The drawing under review shows one solid part. Ordinate dimensions are in mm from its lowest x, y, z. A direction names the side the tool comes from. Give positions to 0.01 mm unless a question says otherwise; leave off trailing zeros. Order: outer loops, then holes, each group sorted by start corner. A loop starts at its lowest first (then second) coordinate and runs counter-clockwise, first axis right, second up. Notation, with made-up numbers: (44, 39) - (102, 39) arc R17 ccw to (102, 51) - close; hole circle Ø9 at (-8, 12). An arc over 180 degrees is marked (long way). Use CSV: the item, a comma, the result in double quotes. Start each with the question number.
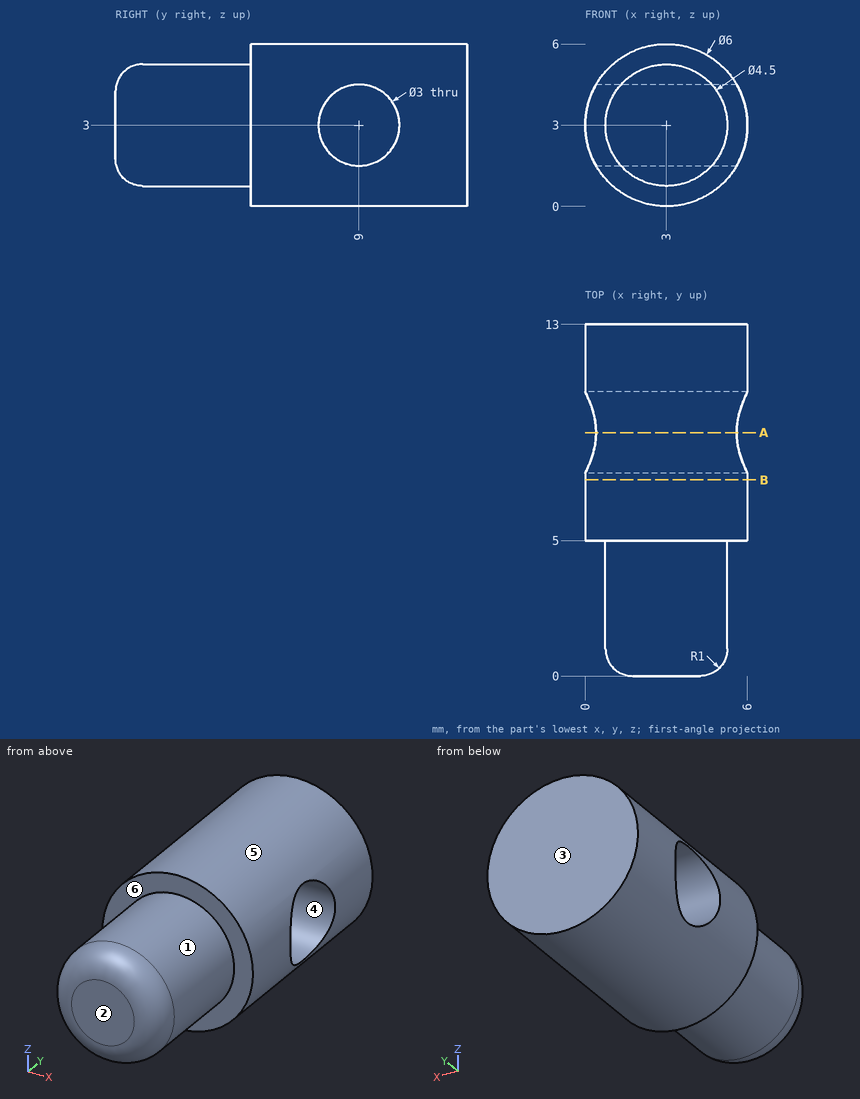
1. Clearance check with flat-ended pins moving along their axes: pin 1 (1 mm diameter, centred on x = 1, y = 6.5, fed in from -Z); pin 2 (2 mm diameter, centred on y = 9, z = 5, fed in from -X); pin 3 (1.5 mm diameter, centred on y = 8, z = 5, fed in from +X). State where each tip first meets the part, or that it passes through.
2. To check wall thickness, follow L1, parallel to Y at x = 3.5, z = 3; L2, parallel to Z at x = 3, y = 9; L3, parallel to X at y = 3, z = 3. State the ranges of each line that lie inside material, in increasing order. Write a range as [from, to].
3. Tool access review of the marked faces 5 and 6: name each direction out of +Z, -Z, +X, -X, +Y, -Y from which nothing blocks a thin tool from reaching the whole face with its end or side.
4. Mouldability with a two-part tool opening along Y and no side actions: class the marked faces 1, 2, 3 and 4 as pulls with the +Y half, pulls with the -Y half, needs draft (parallel to the pull), parting line crosses it, or undercut.
5. Consider section B-B (y = 7.25). Give the boundary of the cut face in (x, z), and give its area (3 significant figures).
6. Consider section A-A (y = 9). Give the boundary of the cut face in (x, z), and give its area (3 significant figures).
Answers follow:
1,pin 1,"stops at z = 0.4"
1,pin 2,"stops at x = 0.3"
1,pin 3,"stops at x = 5.73"
2,L1,"y = [0, 7.5], [10.5, 13]"
2,L2,"z = [0, 1.5], [4.5, 6]"
2,L3,"x = [0.75, 5.25]"
3,face 5,"+Y, -Y"
3,face 6,"-Y"
4,face 1,"needs draft"
4,face 2,"pulls with the -Y half"
4,face 3,"pulls with the +Y half"
4,face 4,"undercut"
5,outline,"circle Ø6 at (3, 3)"
5,area,"28.3 mm^2"
6,outline,"(0.4, 1.5) arc R3 ccw to (5.6, 1.5) - close; (0.4, 4.5) - (5.6, 4.5) arc R3 ccw to start"
6,area,"11.1 mm^2"
